from build123d import *

# Parameters (mm, degrees)
SKETCH1_R      = 1.25
EXTRUDE1_DEPTH = 1
FILLET1_R      = 2


with BuildPart() as part:
    # Sketch1 → Extrude1 (new, symmetric)
    with BuildSketch(Plane(origin=(0, 0, 0), x_dir=(0, 0, -1), z_dir=(1, 0, 0))):
        with BuildLine():
            Line((-0.399660107, 22.896512219), (-0.520081712, 29.795461316))
            ThreePointArc((-0.520081712, 29.795461316), (-6.279068206, 29.1309681), (-11.800426172, 27.364026425))
            Line((-11.800426172, 27.364026425), (-12.910119658, 22.913288948))
            ThreePointArc((-12.910119658, 22.913288948), (0, -28), (12.910119658, 22.913288948))
            Line((12.910119658, 22.913288948), (11.800426172, 27.364026425))
            ThreePointArc((11.800426172, 27.364026425), (6.279068206, 29.1309681), (0.520081712, 29.795461316))
            Line((0.520081712, 29.795461316), (0.399660107, 22.896512219))
            ThreePointArc((0.399660107, 22.896512219), (0, -22.9), (-0.399660107, 22.896512219))
        make_face()
        with Locations((-5.820259343, 26.252420839)):
            Circle(SKETCH1_R, mode=Mode.SUBTRACT)
        with Locations((5.820259343, 26.252420839)):
            Circle(SKETCH1_R, mode=Mode.SUBTRACT)
    extrude(amount=EXTRUDE1_DEPTH, both=True)

    # Fillet1
    fillet1_edges = [part.edges().sort_by_distance(p)[0] for p in [
        (0, 27.364026425, -11.800426172),
        (0, 22.913288948, -12.910119658),
        (0, 22.913288948, 12.910119658),
        (0, 27.364026425, 11.800426172),
    ]]
    fillet(fillet1_edges, radius=FILLET1_R)


solid = part.part
Check sheet for the modelled part. Datum: model origin and axes. Units: mm. Round coordinates to 2 decimals unless told otherwise and drop trailing zeros. Order: outer loops, then holes, each group sorted by start corner. A loop starts at its lowest first (then second) coordinate and runs counter-clockwise, first axis right, second up.
(1) Go/stop test with a flat-tipped pin: P1, Ø2, axis at y = 26.25, z = 5.82, coming from the -X side. Record where the tip stops, or that it passes through.
(2) Cross-section at C-C, the plane y = 0. Enter the section's corners in (x, z), and give its area (3 significant figures).
(3) Scan lines: probe 1 along Y at (x, z) = (-0.45, 0); probe 2 along Y at (x, z) = (0.8, -18.5); probe 3 along Z at (x, y) = (0.4, -15). Record each from-to range of solid material in increasing order.
(4) Cross-section at A-A, the plane y = -21. Enter the section's corners in (x, z).
(5) Draft check along Y on faces 1 (the flat face through (1, -23, -6)), 2 (the cylindrical face through (0.014, 23.024, 13.049)), 3 (the cylindrical face through (0, 27.3, -6.5)). Enter one of: pulls with the +Y half, pulls with the -Y half, needs draft (parallel to the pull), parting line crosses it, or undercut.
(6) Cross-section at B-B, the plane x = -0.65. Enter the section's corners in (y, z), and give its area (3 significant figures).
Check sheet entries:
1. P1: passes through
2. outline: (-1, -27.08) - (1, -27.08) - (1, -22.9) - (-1, -22.9) - close; (-1, 22.9) - (1, 22.9) - (1, 27.08) - (-1, 27.08) - close
2. area: 16.7 mm2
3. probe 1: y = -28 to -22.9
3. probe 2: y = -20.7 to -13.5, 13.5 to 18.89
3. probe 3: z = -23.14 to -17.3, 17.3 to 23.14
4. outline: (-1, -18.17) - (1, -18.17) - (1, -9.13) - (-1, -9.13) - close; (-1, 9.13) - (1, 9.13) - (1, 18.17) - (-1, 18.17) - close
5. face 1: needs draft
5. face 2: pulls with the +Y half
5. face 3: undercut
6. outline: (22.51, -13.64) arc R2 cw to (23.75, -12.7) - (26.38, -12.05) arc R2 ccw to (27.76, -10.83) arc R29.8 ccw to (29.8, -0.52) - (22.9, -0.4) arc R22.9 cw (long way) to (22.9, 0.4) - (29.8, 0.52) arc R29.8 ccw to (27.76, 10.83) arc R2 ccw to (26.38, 12.05) - (23.75, 12.7) arc R2 cw to (22.51, 13.64) arc R27.09 ccw (long way) to start; hole circle Ø2.5 at (26.25, -5.82); hole circle Ø2.5 at (26.25, 5.82)
6. area: 734 mm2
